Can you work these out from the model? Positions are in its coordinate system, mm. Give positions to 0.01 mm unless a question says otherwise; leave off trailing zeros. Order: outer loops, then holes, each group sorted by start corner. A loop starts at its lowest first (then second) coordinate and runs counter-clockwise, first axis right, second up.
Item 1: I want a section at A-A, the plane z = -1. Count the separate pieces of the cut face and the enclosed holes in it, then the cut area to 3 significant figures.
Item 2: I want a section at B-B, the plane y = -102.5. Write out the boundary of the cut face in (x, z).
Item 3: I want a section at C-C, the plane x = 12. Write out the boundary of the cut face in (y, z).
Item 4: If I drill on line 1 along Y through (x, z) = (157.25, -6.1); line 2 along X through (y, z) = (74.5, -5); line 3 along Z through (x, y) = (74, -10), over which ranges is the centre line in solid material (lowest first)?
Item 5: I'm going to push flat-ended pins straight in: pin 1 Ø2.5 at (x, y) = (156.5, -121.5) entering from -Z; pin 2 Ø1 at (x, y) = (157.5, 77) entering from -Z; pin 3 Ø1.6 at (y, z) = (-123, -5) entering from +X; pin 4 Ø2 at (y, z) = (-28.5, -0.5) entering from +X. Where does each tip first touch, or does it pass through?
```python
from build123d import *

# Parameters (mm, degrees)
BOSS_EXTRUDE1_DEPTH = 3
SKETCH2_W           = 166
SKETCH2_H           = 211.014567036
SKETCH2_W_2         = 100
SKETCH2_H_2         = 50
BOSS_EXTRUDE2_DEPTH = 3
CUT_EXTRUDE1_DEPTH  = 3
FILLET1_R           = 5
SKETCH4_W           = 7.5
SKETCH4_H           = 7.5
BOSS_EXTRUDE3_DEPTH = 11
FILLET2_R           = 1
SKETCH5_R           = 1.6
CUT_EXTRUDE2_DEPTH  = 5
SKETCH6_R           = 2.25
CUT_EXTRUDE3_DEPTH  = 3
SKETCH7_W           = 166
SKETCH7_H           = 211.014567036
CUT_EXTRUDE4_DEPTH  = 1


with BuildPart() as part:
    # Sketch1 → Boss-Extrude1 (new body)
    with BuildSketch(Plane.XY):
        with BuildLine():
            Line((48, 73.257283518), (48, -16.742716482))
            ThreePointArc((48, -16.742716482), (50.050252532, -21.69246395), (55, -23.742716482))
            Line((55, -23.742716482), (105, -23.742716482))
            ThreePointArc((105, -23.742716482), (109.949747468, -21.69246395), (112, -16.742716482))
            Line((112, -16.742716482), (112, 73.257283518))
            ThreePointArc((112, 73.257283518), (109.949747468, 78.207030987), (105, 80.257283518))
            Line((105, 80.257283518), (55, 80.257283518))
            ThreePointArc((55, 80.257283518), (50.050252532, 78.207030987), (48, 73.257283518))
        make_face()
        with BuildLine():
            Line((53, 73.257283518), (53, -16.742716482))
            ThreePointArc((53, -16.742716482), (53.585786438, -18.156930044), (55, -18.742716482))
            Line((55, -18.742716482), (105, -18.742716482))
            ThreePointArc((105, -18.742716482), (106.414213562, -18.156930044), (107, -16.742716482))
            Line((107, -16.742716482), (107, 73.257283518))
            ThreePointArc((107, 73.257283518), (106.414213562, 74.671497081), (105, 75.257283518))
            Line((105, 75.257283518), (55, 75.257283518))
            ThreePointArc((55, 75.257283518), (53.585786438, 74.671497081), (53, 73.257283518))
        make_face(mode=Mode.SUBTRACT)
    extrude(amount=-BOSS_EXTRUDE1_DEPTH)

    # Sketch2 → Boss-Extrude2 (add)
    with BuildSketch(Plane.XY):
        with Locations((80, -22.25)):
            Rectangle(SKETCH2_W, SKETCH2_H)
        with Locations((80, 38.257283518)):
            Rectangle(SKETCH2_W_2, SKETCH2_H_2, mode=Mode.SUBTRACT)
    extrude(amount=BOSS_EXTRUDE2_DEPTH)

    # Sketch3 → Cut-Extrude1 (cut)
    with BuildSketch(Plane(origin=(0, 0, -3), x_dir=(-1, 0, 0), z_dir=(0, 0, -1))):
        with BuildLine():
            Line((-55, 80.257283518), (-105, 80.257283518))
            ThreePointArc((-105, 80.257283518), (-109.949747468, 78.207030987), (-112, 73.257283518))
            Line((-112, 73.257283518), (-112, -16.742716482))
            ThreePointArc((-112, -16.742716482), (-109.949747468, -21.69246395), (-105, -23.742716482))
            Line((-105, -23.742716482), (-55, -23.742716482))
            ThreePointArc((-55, -23.742716482), (-50.050252532, -21.69246395), (-48, -16.742716482))
            Line((-48, -16.742716482), (-48, 73.257283518))
            ThreePointArc((-48, 73.257283518), (-50.050252532, 78.207030987), (-55, 80.257283518))
        make_face()
    extrude(amount=-CUT_EXTRUDE1_DEPTH, mode=Mode.SUBTRACT)

    # Fillet1
    fillet1_edges = [part.edges().sort_by_distance(p)[0] for p in [
        (30, 13.257283518, 1.5),
        (130, 13.257283518, 1.5),
        (130, 63.257283518, 1.5),
        (30, 63.257283518, 1.5),
    ]]
    fillet(fillet1_edges, radius=FILLET1_R)

    # Sketch4 → Boss-Extrude3 (add)
    with BuildSketch(Plane.XY.offset(3)):
        with Locations((2.75, 77.507283518)):
            Rectangle(SKETCH4_W, SKETCH4_H)
        with Locations((157.25, -122.007283518)):
            Rectangle(SKETCH4_W, SKETCH4_H)
        with Locations((2.75, -122.007283518)):
            Rectangle(SKETCH4_W, SKETCH4_H)
        with Locations((157.25, 77.507283518)):
            Rectangle(SKETCH4_W, SKETCH4_H)
    extrude(amount=-BOSS_EXTRUDE3_DEPTH)

    # Fillet2
    fillet2_edges = [part.edges().sort_by_distance(p)[0] for p in [
        (-1, 73.757283518, -4),
        (-1, 81.257283518, -4),
        (6.5, 81.257283518, -4),
        (6.5, 73.757283518, -4),
        (161, -118.257283518, -4),
        (161, -125.757283518, -4),
        (153.5, -125.757283518, -4),
        (153.5, -118.257283518, -4),
        (-1, -125.757283518, -4),
        (-1, -118.257283518, -4),
        (6.5, -118.257283518, -4),
        (6.5, -125.757283518, -4),
        (161, 81.257283518, -4),
        (161, 73.757283518, -4),
        (153.5, 73.757283518, -4),
        (153.5, 81.257283518, -4),
    ]]
    fillet(fillet2_edges, radius=FILLET2_R)

    # Sketch5 → Cut-Extrude2 (cut)
    with BuildSketch(Plane(origin=(0, 0, -8), x_dir=(-1, 0, 0), z_dir=(0, 0, -1))):
        with Locations((-157.25, 77.507283518)):
            Circle(SKETCH5_R)
        with Locations((-2.75, 77.507283518)):
            Circle(SKETCH5_R)
        with Locations((-2.75, -122.007283518)):
            Circle(SKETCH5_R)
        with Locations((-157.25, -122.007283518)):
            Circle(SKETCH5_R)
    extrude(amount=-CUT_EXTRUDE2_DEPTH, mode=Mode.SUBTRACT)

    # Sketch6 → Cut-Extrude3 (cut)
    with BuildSketch(Plane(origin=(0, 0, -8), x_dir=(-1, 0, 0), z_dir=(0, 0, -1))):
        with Locations((-157.25, 77.507283518)):
            Circle(SKETCH6_R)
        with Locations((-2.75, 77.507283518)):
            Circle(SKETCH6_R)
        with Locations((-157.25, -122.007283518)):
            Circle(SKETCH6_R)
        with Locations((-2.75, -122.007283518)):
            Circle(SKETCH6_R)
    extrude(amount=-CUT_EXTRUDE3_DEPTH, mode=Mode.SUBTRACT)

    # Sketch7 → Cut-Extrude4 (cut)
    with BuildSketch(Plane(origin=(0, 0, 0), x_dir=(-1, 0, 0), z_dir=(0, 0, -1))):
        with Locations((-80, -22.25)):
            Rectangle(SKETCH7_W, SKETCH7_H)
        with BuildLine():
            Line((-160, 73.757283518), (-154.5, 73.757283518))
            ThreePointArc((-154.5, 73.757283518), (-153.792893219, 74.050176737), (-153.5, 74.757283518))
            Line((-153.5, 74.757283518), (-153.5, 80.257283518))
            ThreePointArc((-153.5, 80.257283518), (-153.792893219, 80.9643903), (-154.5, 81.257283518))
            Line((-154.5, 81.257283518), (-160, 81.257283518))
            ThreePointArc((-160, 81.257283518), (-160.707106781, 80.9643903), (-161, 80.257283518))
            Line((-161, 80.257283518), (-161, 74.757283518))
            ThreePointArc((-161, 74.757283518), (-160.707106781, 74.050176737), (-160, 73.757283518))
        make_face(mode=Mode.SUBTRACT)
        with BuildLine():
            Line((-5.5, 73.757283518), (0, 73.757283518))
            ThreePointArc((0, 73.757283518), (0.707106781, 74.050176737), (1, 74.757283518))
            Line((1, 74.757283518), (1, 80.257283518))
            ThreePointArc((1, 80.257283518), (0.707106781, 80.9643903), (0, 81.257283518))
            Line((0, 81.257283518), (-5.5, 81.257283518))
            ThreePointArc((-5.5, 81.257283518), (-6.207106781, 80.9643903), (-6.5, 80.257283518))
            Line((-6.5, 80.257283518), (-6.5, 74.757283518))
            ThreePointArc((-6.5, 74.757283518), (-6.207106781, 74.050176737), (-5.5, 73.757283518))
        make_face(mode=Mode.SUBTRACT)
        with BuildLine():
            Line((-154.5, -118.257283518), (-160, -118.257283518))
            ThreePointArc((-160, -118.257283518), (-160.707106781, -118.550176737), (-161, -119.257283518))
            Line((-161, -119.257283518), (-161, -124.757283518))
            ThreePointArc((-161, -124.757283518), (-160.707106781, -125.464390299), (-160, -125.757283518))
            Line((-160, -125.757283518), (-154.5, -125.757283518))
            ThreePointArc((-154.5, -125.757283518), (-153.792893219, -125.464390299), (-153.5, -124.757283518))
            Line((-153.5, -124.757283518), (-153.5, -119.257283518))
            ThreePointArc((-153.5, -119.257283518), (-153.792893219, -118.550176737), (-154.5, -118.257283518))
        make_face(mode=Mode.SUBTRACT)
        with BuildLine():
            Line((-6.5, -119.257283518), (-6.5, -124.757283518))
            ThreePointArc((-6.5, -124.757283518), (-6.207106781, -125.464390299), (-5.5, -125.757283518))
            Line((-5.5, -125.757283518), (0, -125.757283518))
            ThreePointArc((0, -125.757283518), (0.707106781, -125.464390299), (1, -124.757283518))
            Line((1, -124.757283518), (1, -119.257283518))
            ThreePointArc((1, -119.257283518), (0.707106781, -118.550176737), (0, -118.257283518))
            Line((0, -118.257283518), (-5.5, -118.257283518))
            ThreePointArc((-5.5, -118.257283518), (-6.207106781, -118.550176737), (-6.5, -119.257283518))
        make_face(mode=Mode.SUBTRACT)
    extrude(amount=-CUT_EXTRUDE4_DEPTH, mode=Mode.SUBTRACT)


solid = part.part
```
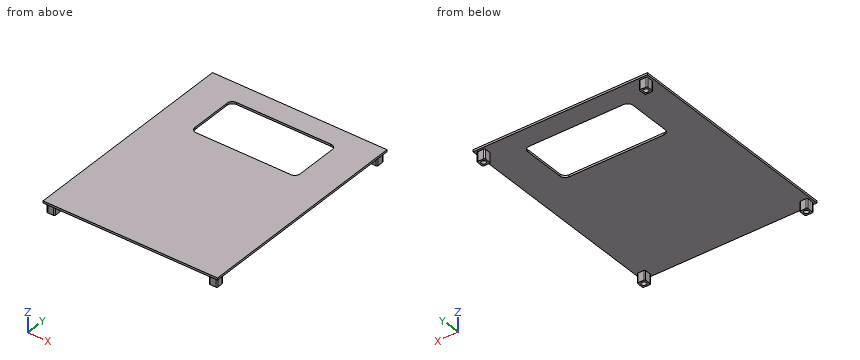
Results list:
1. separate pieces: 4
1. enclosed holes: 0
1. area: 222 mm2
2. outline: (-3, 1) - (163, 1) - (163, 3) - (-3, 3) - close
3. outline: (-127.76, 1) - (83.26, 1) - (83.26, 3) - (-127.76, 3) - close
4. line 1: y = -125.76 to -124.26, -119.76 to -118.26, 73.76 to 75.26, 79.76 to 81.26
4. line 2: x = -0.97 to 6.47, 153.53 to 160.97
4. line 3: z = 1 to 3
5. pin 1: stops at z = -5
5. pin 2: stops at z = -3
5. pin 3: stops at x = 161
5. pin 4: passes through
